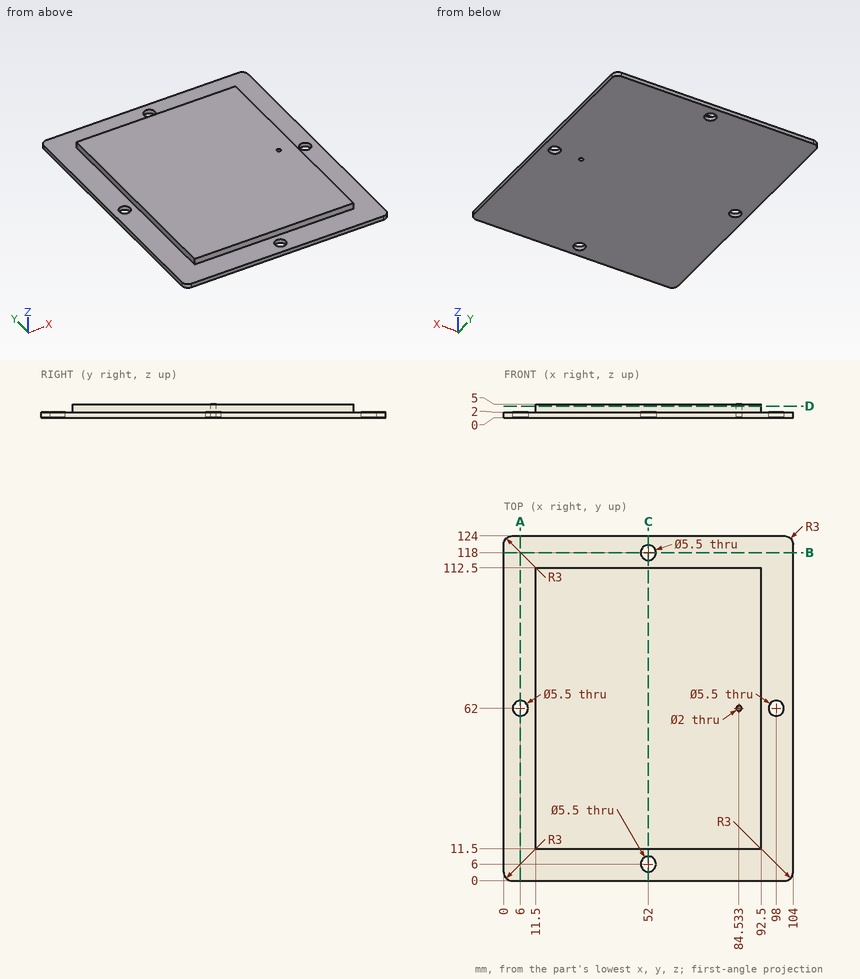
Input: dimensioned drawing with shaded views. Units: mm. Origin: part minimum x, y, z. Coordinates: 2 decimals unless noted, no trailing zeros. Loops run counter-clockwise (first coordinate to the right, second up) from the corner with the lowest first, then second, coordinate; pieces in that order, holes last. Notation, with made-up numbers: M 80.5,78.5 L 109.5,78.5 A19 cw 109.5,115.5 Z; hole C 82,13.5 d8. An arc over 180 degrees is marked long. Use a Markdown table: item, result. Add a question column.
Q1. Section query D-D, the plane z = 4.25. Return loops of the section in (x, y).
Q2. Section query C-C, the plane x = 52. Return loops of the section in (y, z).
Q3. First-contact query: pin 1 (5 mm diameter, centred on x = 52, y = 118, fed in from -Z); pin 2 (0.9 mm diameter, centred on x = 38.5, z = 3.5, fed in from +Y); pin 3 (6.5 mm diameter, centred on x = 98, y = 62, fed in from +Z); pin 4 (1.5 mm diameter, centred on x = 42.5, z = 3.5, fed in from -Y). Flat tips, straight axial feed; report the tip coordinate or a pass-through.
Q4. Section query B-B, the plane y = 118. Return loops of the section in (x, z), and give its area (3 significant figures).
Q5. Section query A-A, the plane x = 6. Return loops of the section in (y, z).
Q6. Material intervals for L1, parallel to Y at x = 52, z = 0.9; L2, parallel to Y at x = 98, z = 0.65; L3, parallel to Z at x = 93.5, y = 19.5, sorted ascending.
Result:
| question | item | result |
|---|---|---|
| 1 | outline | M 11.5,11.5 L 92.5,11.5 L 92.5,112.5 L 11.5,112.5 Z; hole C 84.53,62 d2 |
| 2 | outline | M 0,0 L 3.25,0 L 3.25,2 L 0,2 Z; M 8.75,0 L 115.25,0 L 115.25,2 L 112.5,2 L 112.5,5 L 11.5,5 L 11.5,2 L 8.75,2 Z; M 120.75,0 L 124,0 L 124,2 L 120.75,2 Z |
| 3 | pin 1 | passes through |
| 3 | pin 2 | stops at y = 112.5 |
| 3 | pin 3 | stops at z = 2 |
| 3 | pin 4 | stops at y = 11.5 |
| 4 | outline | M 0,0 L 49.25,0 L 49.25,2 L 0,2 Z; M 54.75,0 L 104,0 L 104,2 L 54.75,2 Z |
| 4 | area | 197 mm2 |
| 5 | outline | M 0,0 L 59.25,0 L 59.25,2 L 0,2 Z; M 64.75,0 L 124,0 L 124,2 L 64.75,2 Z |
| 6 | L1 | y = 0 to 3.25, 8.75 to 115.25, 120.75 to 124 |
| 6 | L2 | y = 0 to 59.25, 64.75 to 124 |
| 6 | L3 | z = 0 to 2 |
